```python
from build123d import *

# Parameters (mm, degrees)
BOSS_EXTRUDE1_DEPTH     = 50.8
CUT_EXTRUDE1_DEPTH      = 50.8
CUT_EXTRUDE1_DEPTH_BACK = 50.8
SKETCH2_R               = 15.875


with BuildPart() as part:
    # Sketch1 → Boss-Extrude1 (new body)
    with BuildSketch(Plane(origin=(0, 0, 0), x_dir=(1, 0, 0), z_dir=(0, 1, 0))):
        with BuildLine():
            Line((-1, 15.968719423), (-1, 12.961481397))
            ThreePointArc((-1, 12.961481397), (0, -13), (1, 12.961481397))
            Line((1, 12.961481397), (1, 15.968719423))
            ThreePointArc((1, 15.968719423), (0, -16), (-1, 15.968719423))
        make_face()
    extrude(amount=BOSS_EXTRUDE1_DEPTH)

    # Sketch2 → Cut-Extrude1 (cut, two sides: drawn at the far end of the back side and taken through both)
    with BuildSketch(Plane.XY.offset(-CUT_EXTRUDE1_DEPTH_BACK)):
        with Locations((0, -9.398568911)):
            Circle(SKETCH2_R)
    extrude(amount=CUT_EXTRUDE1_DEPTH + CUT_EXTRUDE1_DEPTH_BACK, mode=Mode.SUBTRACT)


solid = part.part
```
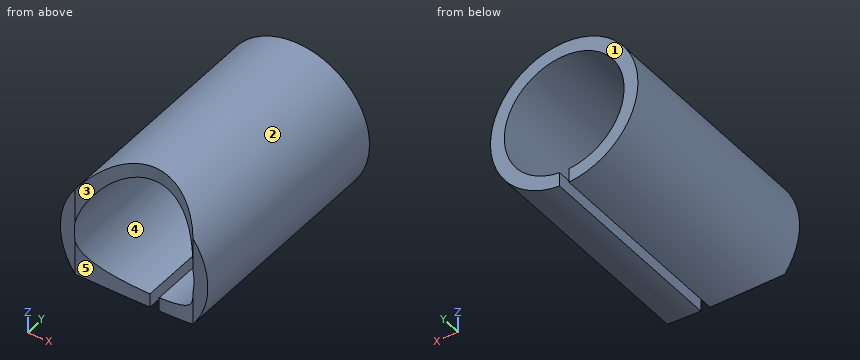
CAD build for the part. Positions are in the model's coordinates, mm. Face numbers are marked on the shaded views. A direction names the side the tool comes from. Coordinates: 2 decimals unless noted, no trailing zeros. Loops run counter-clockwise (first coordinate to the right, second up) from the corner with the lowest first, then second, coordinate; pieces in that order, holes last. Notation, with made-up numbers: (-35.5, 40) - (13.5, 40) arc R17 cw to (13.5, 48) - close; hole circle Ø11 at (53, 61.25). An arc over 180 degrees is marked (long way). Return JSON: item names as keys, results as strings.
1. Band-saw the part on C-C (y = 45.5). Give the cut face in (x, z), and give its area (3 significant figures).
Result:
{"outline": "(-1, -15.97) - (-1, -12.96) arc R13 cw (long way) to (1, -12.96) - (1, -15.97) arc R16 ccw (long way) to start", "area": "267 mm2"}
2. Band-saw the part on D-D (z = -5). Give the cut face in (x, y) (3 decimals), and give its area (3 significant figures).
Result:
{"outline": "(-15.199, 0) - (-12.794, 0) arc R15.875 cw to (-12, 0.994) - (-12, 50.8) - (-15.199, 50.8) - close; (12, 0.994) arc R15.875 cw to (12.794, 0) - (15.199, 0) - (15.199, 50.8) - (12, 50.8) - close", "area": "324 mm2"}
3. 3-axis set-ups, long thin cutter, end or side, ignore diameter. For the marked faces 4 and 5: which of +Z, -Z, +X, -X, +Y, -Y reach the whole face in a straight line?
Result:
{"face 4": "+Y, -Y", "face 5": "+Z, -Z, -Y"}
4. Probe L1, parallel to X at y = 35.5, z = 0; L2, parallel to Z at x = 0, y = 17; L3, parallel to X at y = 32, z = -4.5. List the from-to ranges inside material, lowest first. Write a range as from..to.
Result:
{"L1": "x = -16..-13, 13..16", "L2": "z = 13..16", "L3": "x = -15.35..-12.2, 12.2..15.35"}
5. Band-saw the part on B-B (x = -11.5). Give the cut face in (y, z).
Result:
{"outline": "(1.55, -11.12) - (50.8, -11.12) - (50.8, -6.06) - (1.55, -6.06) - close; (1.55, 6.06) - (50.8, 6.06) - (50.8, 11.12) - (1.55, 11.12) - close"}
6. Drop flat-ended pins along their axis: pin 1 (10 mm diameter, centred on x = 6.5, z = 11, fed in from -Y); pin 2 (5 mm diameter, centred on y = 32.5, z = 8.5, fed in from +X); pin 3 (10 mm diameter, centred on x = 7.5, y = 23, fed in from -Z); pin 4 (8 mm diameter, centred on y = 32, z = -2.5, fed in from +X). Give the stop position or say it passes through.
Result:
{"pin 1": "stops at y = 1.55", "pin 2": "stops at x = 14.83", "pin 3": "stops at z = -15.8", "pin 4": "stops at x = 16"}
7. Mould opens along X. For the marked faces 1, 2 and 3 say: released by +X, released by -X, zero draft, split by the parting line, or undercut.
Result:
{"face 1": "zero draft", "face 2": "split by the parting line", "face 3": "undercut"}
8. Band-saw the part on A-A (z = 11.5). Give the cut face in (x, y) (3 decimals).
Result:
{"outline": "(-11.124, 1.927) arc R15.875 cw to (-6.062, 5.273) - (-6.062, 50.8) - (-11.124, 50.8) - close; (6.062, 5.273) arc R15.875 cw to (11.124, 1.927) - (11.124, 50.8) - (6.062, 50.8) - close"}
